from build123d import *

# Parameters (mm, degrees)
F0_W      = 28.2
F0_H      = 21
F1_DEPTH  = 4
F3_DEPTH  = 2.2
F5_R      = 0.875
F6_DEPTH  = 25
F7_W      = 20.5
F7_H      = 4.5
F8_DEPTH  = 27.5
F9_R      = 1.575
F10_DEPTH = 29
F11_W     = 21
F11_H     = 1
F12_DEPTH = 28.2
F13_W     = 23
F13_H     = 4.5
F14_DEPTH = 3.5
F15_DEPTH = 3
F16_W     = 11
F16_H     = 1.75
F17_DEPTH = 1.85
F18_W     = 21.7
F18_H     = 8
F19_DEPTH = 1.85


# Not quite as in the source:
# - a feature names something its author has since deleted; it is built from what else it names


with BuildPart() as f1:
    # F0 (on Top) → F1 (new body, symmetric)
    with BuildSketch(Plane.XY):
        Rectangle(F0_W, F0_H)
    extrude(amount=F1_DEPTH, both=True)

    # F2 (on face) → F3 (cut)
    with BuildSketch(Plane.XY.offset(4)):
        with BuildLine():
            Line((10.25, 7.75), (-10.25, 7.75))
            Line((-10.25, 7.75), (-10.25, 2.5))
            ThreePointArc((-10.25, 2.5), (-8.482233047, 1.767766953), (-7.75, 0))
            ThreePointArc((-7.75, 0), (-8.482233047, -1.767766953), (-10.25, -2.5))
            Line((-10.25, -2.5), (-10.25, -7.75))
            Line((-10.25, -7.75), (10.25, -7.75))
            Line((10.25, -7.75), (10.25, -2.5))
            ThreePointArc((10.25, -2.5), (7.75, 0), (10.25, 2.5))
            Line((10.25, 2.5), (10.25, 7.75))
        make_face()
        with BuildLine():
            ThreePointArc((-7.75, 0), (-8.482233047, 1.767766953), (-10.25, 2.5))
            Line((-10.25, 2.5), (-10.25, -2.5))
            ThreePointArc((-10.25, -2.5), (-8.482233047, -1.767766953), (-7.75, 0))
        make_face()
        with BuildLine():
            Line((-10.25, -2.5), (-10.25, 2.5))
            ThreePointArc((-10.25, 2.5), (-12.75, 0), (-10.25, -2.5))
        make_face()
        with BuildLine():
            ThreePointArc((12.75, 0), (12.017766953, 1.767766953), (10.25, 2.5))
            Line((10.25, 2.5), (10.25, -2.5))
            ThreePointArc((10.25, -2.5), (12.017766953, -1.767766953), (12.75, 0))
        make_face()
        with BuildLine():
            Line((10.25, -2.5), (10.25, 2.5))
            ThreePointArc((10.25, 2.5), (7.75, 0), (10.25, -2.5))
        make_face()
    extrude(amount=-F3_DEPTH, mode=Mode.SUBTRACT)

    # F5 (on face) → F6 (cut)
    with BuildSketch(Plane.XY.offset(4)):
        with Locations((-12.25, 8.2)):
            Circle(F5_R)
        with Locations((12.25, 8.2)):
            Circle(F5_R)
        with Locations((12.25, -8.2)):
            Circle(F5_R)
        with Locations((-12.25, -8.2)):
            Circle(F5_R)
    extrude(amount=-F6_DEPTH, mode=Mode.SUBTRACT)

    # F7 (on Top) → F8 (cut, symmetric)
    with BuildSketch(Plane.XY):
        with Locations((0, 4.37)):
            Rectangle(F7_W, F7_H)
    extrude(amount=F8_DEPTH, both=True, mode=Mode.SUBTRACT)

    # F9 (on face) → F10 (cut)
    with BuildSketch(Plane.YZ.offset(14.1)):
        with Locations((-3.925, 0)):
            Circle(F9_R)
    extrude(amount=-F10_DEPTH, mode=Mode.SUBTRACT)

    # F11 (on face) → F12 (cut)
    with BuildSketch(Plane.YZ.offset(14.1)):
        with Locations((0, -3.5)):
            Rectangle(F11_W, F11_H)
    extrude(amount=-F12_DEPTH, mode=Mode.SUBTRACT)

    # F13 (on face) → F14 (cut)
    with BuildSketch(Plane.XY.offset(4)):
        with Locations((0, 4.37)):
            Rectangle(F13_W, F13_H)
    extrude(amount=-F14_DEPTH, mode=Mode.SUBTRACT)

    # F13 (on face) → F15 (cut)
    with BuildSketch(Plane.XY.offset(4)):
        with Locations((0, 4.37)):
            Rectangle(F13_W, F13_H)
    extrude(amount=-F15_DEPTH, mode=Mode.SUBTRACT)

    # F16 (on face) → F17 (cut)
    with BuildSketch(Plane.XY.offset(4)):
        with Locations((5.1, 8.625)):
            Rectangle(F16_W, F16_H)
    extrude(amount=-F17_DEPTH, mode=Mode.SUBTRACT)

    # F18 (on face) → F19 (cut)
    with BuildSketch(Plane.XY.offset(4)):
        with Locations((-0.25, -5.5)):
            Rectangle(F18_W, F18_H)
    extrude(amount=-F19_DEPTH, mode=Mode.SUBTRACT)


solid = f1.part
Source: CAD feature listing. Evaluate the final solid. Frame: model axes, mm. A direction names the side the tool comes from. Round coordinates to 2 decimals unless told otherwise and drop trailing zeros. Loops run counter-clockwise (first coordinate to the right, second up) from the corner with the lowest first, then second, coordinate; pieces in that order, holes last. Notation, with made-up numbers: M 1.25,34 L 25.25,34 A26 ccw 25.25,48 Z; hole C 65.5,50.5 d6. An arc over 180 degrees is marked long. Return JSON: item names as keys, results as strings. Group by question number.
1. Section query D-D on z = -2.25. Output: boundary loops of the cut face in (x, y) (3 decimals), and give its area (3 significant figures).
2. Reachability of faces 4 (the face through (11.556, -8.732, 0.549)), 5 (the face through (-1, -8, 2.15)) from +Z, -Z, +X, -X, +Y, -Y: full face, straight path, thin tool, end or side. Return the list, or none.
3. Mould query, pull axis X, two halves, no side actions, for faces 1 (the face through (14.1, 0, 1)), 2 (the face through (11, 4, 0.5)), 3 (the face through (0, 10.5, 1)). Classes: released by +X, released by -X, zero draft, split by the parting line, or undercut.
4. Section query B-B on z = 0. Output: boundary loops of the cut face in (x, y) (3 decimals), and give its area (4 significant figures).
5. Material intervals for line 1 along X through (y, z) = (5.5, -1.5); line 2 along Y through (x, z) = (12.25, 0.5) (3 decimals); line 3 along Y through (x, z) = (12.25, -0.25) (3 decimals), sorted ascending. Write a range as from..to.
6. Pin query (flat end, axial travel): pin 1 (4 mm diameter, centred on x = 7, y = 2, fed in from +Z); pin 2 (1.6 mm diameter, centred on x = 12.25, y = -8.2, fed in from +Z); pin 3 (1.5 mm diameter, centred on x = -1.5, y = -8, fed in from +Z). Return the tip coordinate at first contact, or that it passes through.
7. Section query A-A on x = 5.25. Output: boundary loops of the cut face in (y, z) (3 decimals).
8. Section query C-C on x = -12.25. Output: boundary loops of the cut face in (y, z) (3 decimals), and give its area (3 significant figures).
Checks:
{
 "1": {"outline": "M -14.1,-10.5 L 14.1,-10.5 L 14.1,10.5 L -14.1,10.5 Z; hole C -12.25,-8.2 d1.75; hole C -12.25,8.2 d1.75; hole M -10.25,2.12 L 10.25,2.12 L 10.25,6.62 L -10.25,6.62 Z; hole C 12.25,-8.2 d1.75; hole C 12.25,8.2 d1.75", "area": "490 mm²"},
 "2": {"face 4": "+Z, -Z", "face 5": "+Z"},
 "3": {"face 1": "released by +X", "face 2": "undercut", "face 3": "zero draft"},
 "4": {"outline": "M -14.1,-10.5 L 14.1,-10.5 L 14.1,-5.5 L -14.1,-5.5 Z; M -14.1,-2.35 L 14.1,-2.35 L 14.1,10.5 L -14.1,10.5 Z; hole C -12.25,-8.2 d1.75; hole C -12.25,8.2 d1.75; hole M -10.25,2.12 L 10.25,2.12 L 10.25,6.62 L -10.25,6.62 Z; hole C 12.25,-8.2 d1.75; hole C 12.25,8.2 d1.75", "area": "401.5 mm²"},
 "5": {"line 1": "x = -14.1..-10.25, 10.25..14.1", "line 2": "y = -10.5..-9.075, -7.325..-5.419, -2.431..7.325, 9.075..10.5", "line 3": "y = -10.5..-9.075, -7.325..-5.48, -2.37..7.325, 9.075..10.5"},
 "6": {"pin 1": "stops at z = 1.8", "pin 2": "passes through", "pin 3": "stops at z = 2.15"},
 "7": {"outline": "M -10.5,-3 L 2.12,-3 L 2.12,1.8 L -7.75,1.8 L -7.75,2.15 L -9.5,2.15 L -9.5,4 L -10.5,4 Z; M 6.62,-3 L 10.5,-3 L 10.5,4 L 9.5,4 L 9.5,2.15 L 7.75,2.15 L 7.75,1.8 L 6.62,1.8 Z; hole C -3.925,0 d3.15"},
 "8": {"outline": "M -10.5,-3 L -9.075,-3 L -9.075,4 L -10.5,4 Z; M -7.325,-3 L 7.325,-3 L 7.325,4 L 1.5,4 L 1.5,1.8 L -1.5,1.8 L -1.5,4 L -7.325,4 Z; M 9.075,-3 L 10.5,-3 L 10.5,4 L 9.075,4 Z; hole C -3.925,0 d3.15", "area": "108 mm²"}
}
